Verification items for the finished model (mm, model axes). A direction names the side the tool comes from. Coordinates: 2 decimals unless noted, no trailing zeros. Order: outer loops, then holes, each group sorted by start corner. A loop starts at its lowest first (then second) coordinate and runs counter-clockwise, first axis right, second up. Notation, with made-up numbers: (28, 45.5) - (48, 45.5) arc R20 cw to (48, 69.5) - close; hole circle Ø5 at (37.5, 3.25). An arc over 180 degrees is marked (long way). Answer as CSV lines item,"result". Start each with the question number.
1. Go/stop test with a flat-tipped pin: pin 1 (3 mm diameter, centred on x = 29.5, z = -8, fed in from -Y). Record where the tip stops, or that it passes through.
2. Section check B-B (z = 0). Record the cut outline in (x, y), and give its area (3 significant figures).
3. Set-up check for faces 4 (the flat face through (-1, -7, -26)), 5 (the flat face through (57, -5, 0)): record each of +Z, -Z, +X, -X, +Y, -Y from which the full face is reachable in a straight line by a thin tool's end or side.
4. Section check A-A (y = -8.25). Record the cut outline in (x, z), and give its area (3 significant figures).
5. Section check C-C (x = 2). Record the cut outline in (y, z), and give its area (3 significant figures).
6. Material ranges on L1, parallel to Z at x = -12, y = -7; L2, parallel to X at y = -7.75, z = -22; L3, parallel to Y at x = 27, z = -5.5, recorded low to high. Write a range as [from, to].
7. Mould release check, pull along Z, two halves, no side actions. Record for faces 1 (the flat face through (-1, -5, -32)), 2 (the flat face through (-4.5, -10, 26.2)), 3 (the flat face through (-1, -7, 26)): pulls with the +Z half, pulls with the -Z half, needs draft (parallel to the pull), parting line crosses it, or undercut.
from build123d import *

# Parameters (mm, degrees)
F0_W     = 114
F0_H     = 64
F1_DEPTH = 5
F2_W     = 114
F2_H     = 64
F2_W_2   = 102
F2_H_2   = 52
F3_DEPTH = 5


with BuildPart() as f1:
    # F0 (on Front) → F1 (new body)
    with BuildSketch(Plane.XZ):
        Rectangle(F0_W, F0_H)
    extrude(amount=F1_DEPTH)

    # F2 (on face) → F3 (join)
    with BuildSketch(Plane.XZ.offset(5)):
        Rectangle(F2_W, F2_H)
        Rectangle(F2_W_2, F2_H_2, mode=Mode.SUBTRACT)
    extrude(amount=F3_DEPTH)


solid = f1.part
Evaluation:
1,pin 1,"stops at y = -5"
2,outline,"(-57, -10) - (-51, -10) - (-51, -5) - (51, -5) - (51, -10) - (57, -10) - (57, 0) - (-57, 0) - close"
2,area,"630 mm²"
3,face 4,"-Y"
3,face 5,"+Z, -Z, +X, +Y, -Y"
4,outline,"(-57, -32) - (57, -32) - (57, 32) - (-57, 32) - close; hole (-51, -26) - (51, -26) - (51, 26) - (-51, 26) - close"
4,area,"1,990 mm²"
5,outline,"(-10, -32) - (0, -32) - (0, 32) - (-10, 32) - (-10, 26) - (-5, 26) - (-5, -26) - (-10, -26) - close"
5,area,"380 mm²"
6,L1,"z = [-32, -26], [26, 32]"
6,L2,"x = [-57, -51], [51, 57]"
6,L3,"y = [-5, 0]"
7,face 1,"pulls with the -Z half"
7,face 2,"needs draft"
7,face 3,"undercut"
